Autodesk Inventor part; units mm, degrees
ref_plane "YZ Plane" through (0, 0, 0) normal (1, 0, 0) x (0, 1, 0)
ref_plane "XZ Plane" through (0, 0, 0) normal (0, 1, 0) x (-1, 0, 0)
ref_plane "XY Plane" through (0, 0, 0) normal (0, 0, 1) x (1, 0, 0)
sketch "草圖1" plane through (0, 0, 0) normal (0, 0, 1) x (1, 0, 0)
  line L0 (-1.8649, 0) -> (-1.8649, -6) construction
  line L1 (-1.8649, -6) -> (-0.9249, -6) construction
  line L2 (-1.8649, 0) -> (-1.8649, -6) construction
  line L3 (-0.9249, 0) -> (0, 0)
  line L4 (-0.9249, 0) -> (-0.9249, -6) construction
  line L5 (2.6286, 0) -> (2.6286, -6)
  line L6 (2.6286, -6) -> (7.6286, -6)
  line L7 (7.6286, 0) -> (7.6286, -6)
  line L8 (-1.8949, -3) -> (-0.8949, -3)
  line L9 (-0.8949, -3) -> (-0.8949, -6)
  line L10 (-0.8949, -6) -> (9.1286, -6)
  line L11 (9.1286, -6) -> (9.1286, -7.5)
  line L12 (9.1286, -7.5) -> (-0.3949, -7.5)
  line L13 (-0.3949, -7.5) -> (-0.3949, -20.2) construction
  line L14 (-0.3949, -20.2) -> (-9.8949, -20.2) construction
  line L15 (-9.8949, -20.2) -> (-9.8949, -19)
  line L16 (-9.8949, -19) -> (-1.8949, -19) construction
  line L17 (-1.8949, -6) -> (-9.8949, -6)
  line L18 (-9.8949, -6) -> (-9.8949, -7.5)
  line L19 (-9.8949, -7.5) -> (-0.3949, -7.5)
  line L20 (-1.8949, -19) -> (-1.8949, -7.5) construction
  line L21 (-1.8949, -6) -> (-1.8949, -3)
  dimension "d0" = 1
  dimension "d2" = 1.5
  dimension "d3" = 16
  dimension "d4" = 1.5
  dimension "d6" = 8
  dimension "d7" = 1.2
  dimension "d11" = 3
extrude "擠出1" add sketch "草圖1" along normal blind 6
fillet "圓角1" radius 3 2 edges at (9.1286, -6.75, 6) (9.1286, -6.75, 0)
sketch "草圖2" plane through (-0.8949, -6, 6) normal (0, 1, 0) x (1, 0, 0)
  circle A0 centre (4.97, 3) radius 1.5
  point P0 (0.8949, 6)
extrude "擠出2" [suppressed]
sketch "草圖3" plane through (-9.8949, -7.5, 0) normal (-1, 0, 0) x (0, 0, 1)
  line L0 (0, 1.5) -> (0, 0)
  line L1 (0, 0) -> (6, 0)
  line L2 (6, 1.5) -> (6, 0)
  line L3 (0, 1.5) -> (6, 1.5)
  line L4 (3, 0) -> (3, -6.212)
  line L5 (3, -6.212) -> (0.8685, -6.212)
  line L6 (0.8685, -6.212) -> (0.8685, -7.3106)
  line L7 (0.8685, -7.3106) -> (6, -7.3106)
  line L8 (6, -7.3106) -> (6, 0)
  point P0 (0, 7.5)
properties part number "j1 endstop block"
Geometry: final body of the model. Coordinates: model frame, mm. A direction names the side the tool comes from. Round coordinates to 2 decimals unless told otherwise and drop trailing zeros. Loops run counter-clockwise (first coordinate to the right, second up) from the corner with the lowest first, then second, coordinate; pieces in that order, holes last. Notation, with made-up numbers: (-24.5, -17.75) -> (22.5, -17.75) arc R23 ccw to (22.5, -3.75) -> close; hole circle Ø2 at (30, -11.75). An arc over 180 degrees is marked (long way). Use one line per item in the form item = value. Start each with the question number.
1) Access query for faces 1 (the flat face through (-1.895, -5, 3)), 2 (the flat face through (-2, -7, 6)), 3 (the flat face through (4, -6, 3)). Directions: +Z, -Z, +X, -X, +Y, -Y. A direction counts if a zero-diameter tool reaches every point of the face in a straight line with its end or side. Return the directions, or none.
2) Section B-B on z = 4.45. Output: boundary loops of the cut face in (x, y), then the cut area to 3 significant figures.
3) Section D-D on z = 3.45. Output: boundary loops of the cut face in (x, y), then the cut area to 3 significant figures.
4) First-contact query: P1, Ø3, axis at x = 4, z = 4.5, coming from the +Y side; P2, Ø1, axis at x = 6.5, y = -6, coming from the -Z side; P3, Ø0.9, axis at y = -5, z = 3, coming from the +X side. Flat tips, straight axial feed; report the tip coordinate or a pass-through.
5) Section C-C on x = 1. Output: boundary loops of the cut face in (y, z).
6) Line query: L1, parallel to X at y = -4.55, z = 1.4; L2, parallel to Y at x = 8, z = 4.2; L3, parallel to X at y = -6.9, z = 5.35. Output: solid intervals per line, ascending.
Response:
q1.face_1 = +Z, -Z, -X, +Y
q1.face_2 = +Z, +X, -X, +Y, -Y
q1.face_3 = +Z, -Z, +X, +Y
q2.outline = (-9.89, -7.5) -> (8.76, -7.5) -> (8.76, -6) -> (-0.89, -6) -> (-0.89, -3) -> (-1.89, -3) -> (-1.89, -6) -> (-9.89, -6) -> close
q2.area = 31.0 mm^2
q3.outline = (-9.89, -7.5) -> (9.09, -7.5) -> (9.09, -6) -> (-0.89, -6) -> (-0.89, -3) -> (-1.89, -3) -> (-1.89, -6) -> (-9.89, -6) -> close
q3.area = 31.5 mm^2
q4.P1 = -6
q4.P2 = 0
q4.P3 = -0.89
q5.outline = (-7.5, 0) -> (-6, 0) -> (-6, 6) -> (-7.5, 6) -> close
q6.L1 = -1.89 to -0.89
q6.L2 = -7.5 to -6
q6.L3 = -9.89 to 7.99
